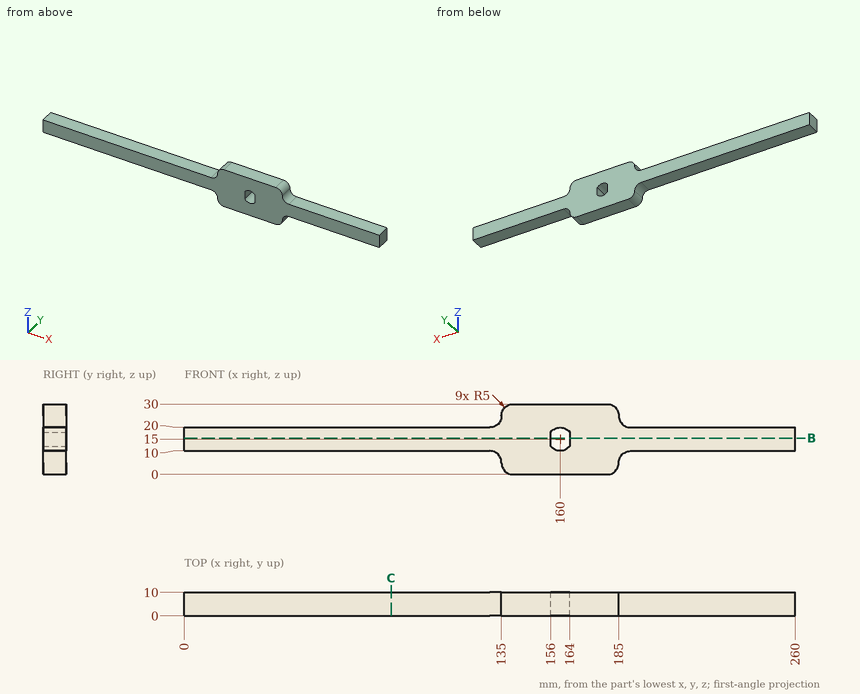
Answer from the drawing. Dimensions are ordinates in mm from the lowest x, y and z of the part. Give positions to 0.01 mm unless a question says otherwise; leave off trailing zeros. Loops run counter-clockwise (first coordinate to the right, second up) from the corner with the lowest first, then second, coordinate; pieces in that order, holes last. Notation, with made-up numbers: M 38,48.5 L 45,48.5 A14 ccw 45,52.5 Z; hole C -38.5,-25.5 d8. An arc over 180 degrees is marked long. One line per item, written item: value.
Q1. A cutting plane is placed at C-C on x = 88. Determine the outline of the cut face in (y, z), then the cut area to 3 significant figures.
Working result:
outline: M 0,10 L 10,10 L 10,20 L 0,20 Z
area: 100 mm^2
Q2. A cutting plane is placed at B-B on z = 15.5. Determine the outline of the cut face in (x, y).
Working result:
outline: M 0,0 L 156,0 L 156,10 L 0,10 Z; M 164,0 L 260,0 L 260,10 L 164,10 Z
Q3. Find the intervals of material crossed by line 1 (X direction, y = 8.5, z = 13.75); line 2 (Z direction, x = 17.5, y = 4.25); line 3 (X direction, y = 6, z = 11.5), in increasing order. Write a range as from..to.
Working result:
line 1: x = 0..156, 164..260
line 2: z = 10..20
line 3: x = 0..156.43, 163.57..260
Q4. Flat-ended cylindrical pins translate along their axes: P1, Ø1, axis at x = 57, y = 5.5, coming from the +Z side; P2, Ø1.5, axis at y = 7.5, z = 4.5, coming from the -X side; P3, Ø1.5, axis at y = 5, z = 24, coming from the -X side. Find the tip coordinate at first contact, or state that the pin passes through.
Working result:
P1: stops at z = 20
P2: stops at x = 134.99
P3: stops at x = 134.68
